Here's how the part is built. I have some questions about the finished solid (model axes, mm). Face numbers are marked on the shaded views. A direction names the side the tool comes from. Round coordinates to 2 decimals unless told otherwise and drop trailing zeros. Loops run counter-clockwise (first coordinate to the right, second up) from the corner with the lowest first, then second, coordinate; pieces in that order, holes last. Notation, with made-up numbers: M 10.5,47.5 L 63.5,47.5 A17 ccw 63.5,59.5 Z; hole C 51,6.25 d5. An arc over 180 degrees is marked long. Use a Markdown table: item, result.
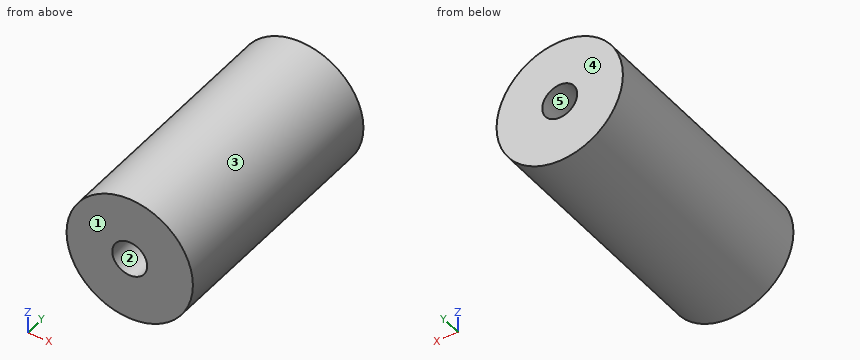
Autodesk Inventor part; units mm, degrees
ref_plane "YZ Plane" through (0, 0, 0) normal (1, 0, 0) x (0, 1, 0)
ref_plane "XZ Plane" through (0, 0, 0) normal (0, 1, 0) x (-1, 0, 0)
ref_plane "XY Plane" through (0, 0, 0) normal (0, 0, 1) x (1, 0, 0)
sketch "Szkic1" plane through (0, 0, 0) normal (0, 1, 0) x (-1, 0, 0)
  circle A0 centre (0, 0) radius 25
extrude "Wyciągnięcie proste1" add sketch "Szkic1" along normal blind 100
sketch "Szkic2" plane through (0, 0, 0) normal (0, -1, 0) x (1, 0, 0)
  circle A0 centre (0, 0) radius 25
hole "Otwór1" at (0, 0, 0) direction (0, 1, 0) diameter 13.835 depth 41.3 tip angle 118
sketch "Szkic3" plane through (0, 100, 0) normal (0, 1, 0) x (1, 0, 0)
  line L0 (0, 0) -> (-13.3904, -21.1115)
  circle A0 centre (0, 0) radius 25
hole "Otwór2" at (0, 100, 0) direction (0, -1, 0) diameter 13.835 depth 41.3 tip angle 118
properties part number "mocowanie_pod_hak"
Q1. Imagine slicing it at B-B, the plane x = -10. Please give me the cut outline in (y, z).
Return value:
| item | result |
|---|---|
| outline | M 0,-22.91 L 100,-22.91 L 100,22.91 L 0,22.91 Z |
Q2. Will these pins go through, and if not, where does the flat tip stop? P1, Ø12, axis at y = 54.5, z = -16.5, coming from the +X side; P2, Ø1.5, axis at y = 39, z = 16.5, coming from the -X side; P3, Ø8, axis at y = 25, z = 17.5, coming from the -X side.
Return value:
| item | result |
|---|---|
| P1 | stops at x = 22.69 |
| P2 | stops at x = -19.41 |
| P3 | stops at x = -21.04 |
Q3. Imagine slicing it at C-C, the plane z = 16. Please give me the cut outline in (x, y).
Return value:
| item | result |
|---|---|
| outline | M -19.21,0 L 19.21,0 L 19.21,100 L -19.21,100 Z |
Q4. For the marked faces 1 and 2, which set-ups out of +Z, -Z, +X, -X, +Y, -Y let a thin tool reach every point of the face, with its end or its side?
Return value:
| item | result |
|---|---|
| face 1 | +Z, -Z, +X, -X, -Y |
| face 2 | -Y |
Q5. We'd pull the mould along X, two halves only. Please class the marked faces 3, 4 and 5: pulls with the +X half, pulls with the -X half, needs draft (parallel to the pull), parting line crosses it, or undercut.
Return value:
| item | result |
|---|---|
| face 3 | parting line crosses it |
| face 4 | needs draft |
| face 5 | undercut |
Q6. I need wall thicknesses on line 1 (Z direction, x = 0, y = 79.5); line 2 (Z direction, x = -5.5, y = 45); line 3 (X direction, y = 33, z = -21.5). Which ranges of each line are inside material? Lowest first, please. Write a range as from..to.
Return value:
| item | result |
|---|---|
| line 1 | z = -25..-6.92, 6.92..25 |
| line 2 | z = -24.39..24.39 |
| line 3 | x = -12.76..12.76 |
Q7. Imagine slicing it at A-A, the plane y = 7. Please give me the cut outline in (x, z) (1 decimal).
Return value:
| item | result |
|---|---|
| outline | C 0,0 d50; hole C 0,0 d13.8 |
